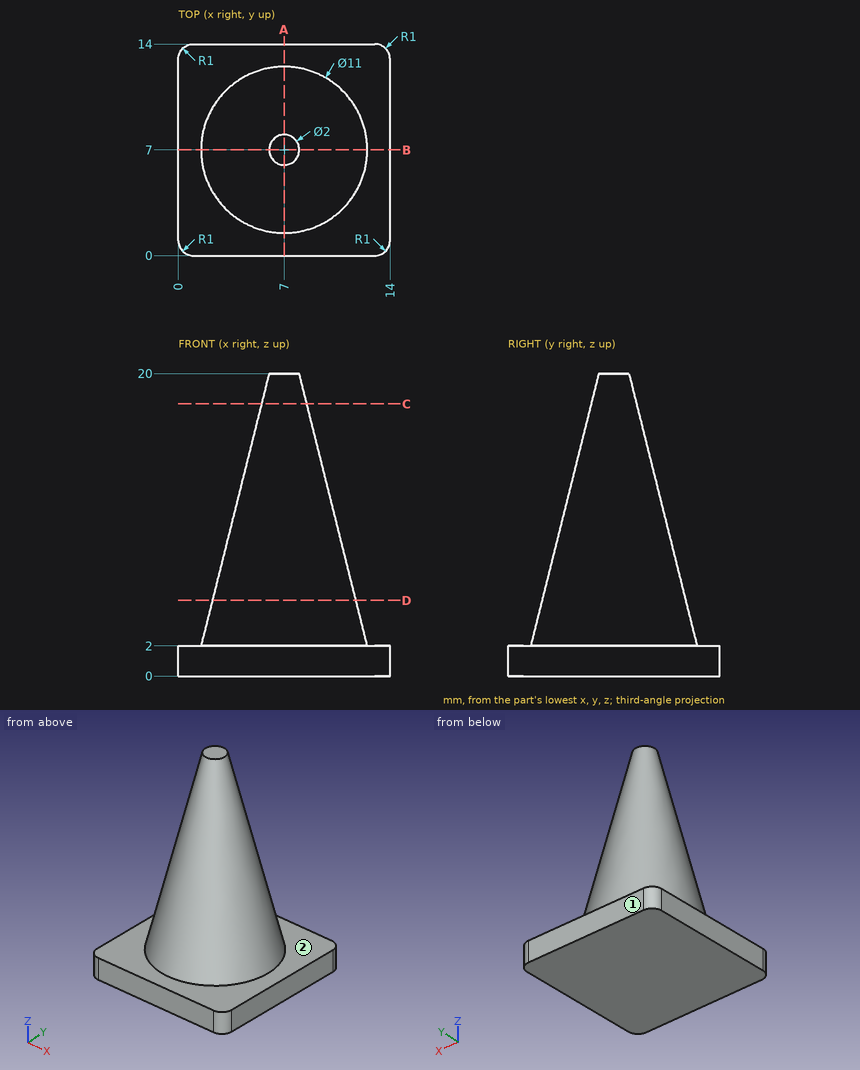
Check sheet for the drawn part. Datum: minimum x, y, z corner. Units: mm. A direction names the side the tool comes from. Round coordinates to 2 decimals unless told otherwise and drop trailing zeros. Order: outer loops, then holes, each group sorted by start corner. A loop starts at its lowest first (then second) coordinate and runs counter-clockwise, first axis right, second up.
(1) Cross-section at A-A, the plane x = 7. Enter the section's corners in (y, z).
(2) Go/stop test with flat-tipped pins: P1, Ø1, axis at y = 4, z = 5, coming from the -X side; P2, Ø6, axis at y = 1.5, z = 10.5, coming from the +X side; P3, Ø8, axis at y = 3, z = 14, coming from the -X side. Record where each tip stops, or that it passes through.
(3) Cross-section at D-D, the plane z = 5. Enter the section's corners in (x, y), and give its area (3 significant figures).
(4) Access from +Z, -Z, +X, -X, +Y, -Y to the whole of each face (thin tool, end or side, straight path). Record for the marked faces 1 and 2.
(5) Scan lines: probe 1 along Z at (x, y) = (1.5, 2.5); probe 2 along X at (y, z) = (2.75, 3); probe 3 along X at (y, z) = (5.5, 9.5). Record each from-to range of solid material in increasing order.
(6) Cross-section at C-C, the plane z = 18. Enter the section's corners in (x, y), and give its area (3 significant figures).
Check sheet entries:
1. outline: (0, 0) - (14, 0) - (14, 2) - (12.5, 2) - (8, 20) - (6, 20) - (1.5, 2) - (0, 2) - close
2. P1: stops at x = 2.93
2. P2: stops at x = 9.45
2. P3: stops at x = 4
3. outline: circle Ø9.5 at (7, 7)
3. area: 70.9 mm2
4. face 1: +Z, -Z, +X, -X, +Y
4. face 2: +Z
5. probe 1: z = 0 to 2
5. probe 2: x = 3.92 to 10.08
5. probe 3: x = 3.7 to 10.3
6. outline: circle Ø3 at (7, 7)
6. area: 7.07 mm2
